from build123d import *

# Parameters (mm, degrees)
SKETCH1_W                = 151
SKETCH1_H                = 84
BOSS_EXTRUDE1_DEPTH      = 37
SKETCH3_W                = 145
SKETCH3_H                = 78
CUT_EXTRUDE3_DEPTH       = 34
SKETCH8_W                = 19
SKETCH8_H                = 14
CUT_EXTRUDE4_DEPTH       = 3
SKETCH9_W                = 19
SKETCH9_H                = 14
CUT_EXTRUDE5_DEPTH       = 3
SKETCH11_W               = 9
SKETCH11_H               = 10
CUT_EXTRUDE6_DEPTH       = 3
SKETCH12_W               = 9
SKETCH12_H               = 10
CUT_EXTRUDE7_DEPTH       = 3
BOSS_EXTRUDE2_DEPTH      = 3
BOSS_EXTRUDE2_DEPTH_BACK = 3
SKETCH19_R               = 1.5
CUT_EXTRUDE8_DEPTH       = 6
SKETCH20_W               = 3
SKETCH20_H               = 14
BOSS_EXTRUDE3_DEPTH      = 3
SKETCH21_W               = 3
SKETCH21_H               = 14
BOSS_EXTRUDE4_DEPTH      = 3
SKETCH23_W               = 16
SKETCH23_H               = 15
CUT_EXTRUDE9_DEPTH       = 3
SKETCH28_W               = 4
SKETCH28_H               = 5
BOSS_EXTRUDE5_DEPTH      = 5
MIRROR2_COPY_1_SKETCH_W  = 4
MIRROR2_COPY_1_SKETCH_H  = 5
MIRROR2_COPY_1_DEPTH     = 5


with BuildPart() as part:
    # Sketch1 → Boss-Extrude1 (new body)
    with BuildSketch(Plane.XY):
        Rectangle(SKETCH1_W, SKETCH1_H)
    extrude(amount=BOSS_EXTRUDE1_DEPTH)

    # Sketch3 → Cut-Extrude3 (cut)
    with BuildSketch(Plane.XY.offset(37)):
        Rectangle(SKETCH3_W, SKETCH3_H)
    extrude(amount=-CUT_EXTRUDE3_DEPTH, mode=Mode.SUBTRACT)

    # Sketch8 → Cut-Extrude4 (cut)
    with BuildSketch(Plane.ZY.offset(75.5)):
        with Locations((27.5, -24)):
            Rectangle(SKETCH8_W, SKETCH8_H)
    extrude(amount=-CUT_EXTRUDE4_DEPTH, mode=Mode.SUBTRACT)

    # Sketch9 → Cut-Extrude5 (cut)
    with BuildSketch(Plane.ZY.offset(75.5)):
        with Locations((27.5, -6)):
            Rectangle(SKETCH9_W, SKETCH9_H)
    extrude(amount=-CUT_EXTRUDE5_DEPTH, mode=Mode.SUBTRACT)

    # Sketch11 → Cut-Extrude6 (cut)
    with BuildSketch(Plane(origin=(75.5, 0, 0), x_dir=(0, 0, -1), z_dir=(1, 0, 0))):
        with Locations((-7.5, 32)):
            Rectangle(SKETCH11_W, SKETCH11_H)
    extrude(amount=-CUT_EXTRUDE6_DEPTH, mode=Mode.SUBTRACT)

    # Sketch12 → Cut-Extrude7 (cut)
    with BuildSketch(Plane(origin=(75.5, 0, 0), x_dir=(0, 0, -1), z_dir=(1, 0, 0))):
        with Locations((-7.5, -26)):
            Rectangle(SKETCH12_W, SKETCH12_H)
    extrude(amount=-CUT_EXTRUDE7_DEPTH, mode=Mode.SUBTRACT)

    # Sketch16 → Boss-Extrude2 (add, two sides)
    with BuildSketch(Plane.XY.offset(18)) as boss_extrude2_sk:
        with BuildLine():
            Line((75.5, 6), (75.5, -8.461119278))
            ThreePointArc((75.5, -8.461119278), (82.730559639, -1.230559639), (75.5, 6))
        make_face()
    extrude(amount=BOSS_EXTRUDE2_DEPTH)
    extrude(boss_extrude2_sk.sketch, amount=-BOSS_EXTRUDE2_DEPTH_BACK)

    # Sketch19 → Cut-Extrude8 (cut)
    with BuildSketch(Plane.XY.offset(21)):
        with Locations((79, -1)):
            Circle(SKETCH19_R)
    extrude(amount=-CUT_EXTRUDE8_DEPTH, mode=Mode.SUBTRACT)

    # Sketch20 → Boss-Extrude3 (add)
    with BuildSketch(Plane.ZY.offset(75.5)):
        with Locations((35.5, -6)):
            Rectangle(SKETCH20_W, SKETCH20_H)
    extrude(amount=-BOSS_EXTRUDE3_DEPTH)

    # Sketch21 → Boss-Extrude4 (add)
    with BuildSketch(Plane.ZY.offset(75.5)):
        with Locations((35.5, -24)):
            Rectangle(SKETCH21_W, SKETCH21_H)
    extrude(amount=-BOSS_EXTRUDE4_DEPTH)

    # Sketch23 → Cut-Extrude9 (cut)
    with BuildSketch(Plane.ZY.offset(75.5)):
        with Locations((26, 10.5)):
            Rectangle(SKETCH23_W, SKETCH23_H)
    extrude(amount=-CUT_EXTRUDE9_DEPTH, mode=Mode.SUBTRACT)

    # Sketch28 → Boss-Extrude5 (add)
    with BuildSketch(Plane.ZY.offset(-72.5)):
        with Locations((32, -36.5)):
            Rectangle(SKETCH28_W, SKETCH28_H)
    boss_extrude5 = extrude(amount=BOSS_EXTRUDE5_DEPTH)

    # Mirror1: Boss-Extrude5 across plane
    add(boss_extrude5.mirror(Plane.ZX))

    # Mirror2: Boss-Extrude5 across plane
    add(boss_extrude5.mirror(Plane(origin=(0, 0, 0), x_dir=(0, 0, 1), z_dir=(1, 0, 0))))

    # Mirror2 copy 1 sketch → Mirror2 copy 1 (add)
    with BuildSketch(Plane(origin=(-72.5, 0, 0), x_dir=(0, 0, 1), z_dir=(1, 0, 0))):
        with Locations((32, -36.5)):
            Rectangle(MIRROR2_COPY_1_SKETCH_W, MIRROR2_COPY_1_SKETCH_H)
    extrude(amount=MIRROR2_COPY_1_DEPTH)


solid = part.part
Design review of the part built by this model. Coordinates are the model's own, in mm. A direction names the side the tool comes from. Round coordinates to 2 decimals unless told otherwise and drop trailing zeros. Loops run counter-clockwise (first coordinate to the right, second up) from the corner with the lowest first, then second, coordinate; pieces in that order, holes last. Notation, with made-up numbers: (-4, 32.5) - (13, 32.5) arc R15 ccw to (13, 41.5) - close; hole circle Ø5 at (70.5, 17.25). An arc over 180 degrees is marked (long way). One line per item, written item: value. Start each with the question number.
1) Consider section A-A on z = 32. Give the boundary of the cut face in (x, y).
2) Consider section C-C on y = -1. Give the boundary of the cut face in (x, z).
3) For faces 1 (the flat face through (-74, -31, 26)), 2 (the flat face through (70, -34, 32)), 3 (the flat face through (70, 37, 30)), list the 3-axis set-ups (+Z, -Z, +X, -X, +Y, -Y) from which the entire face can be reached by the end or side of a thin tool; tool diameter is ignored.
4) To check wall thickness, follow L1, parallel to Y at x = -26, z = 15; L2, parallel to X at y = -38, z = 32; L3, parallel to X at y = 21.5, z = 7. State the ranges of each line that lie inside material, in increasing order. Write a range as from..to.
5) Consider section B-B on x = 69. Give the boundary of the cut face in (y, z), then the cut area to 3 significant figures.
6) Draft analysis for pull direction X (two halves, no side actions). For faces 4 (the flat face through (74, 32, 12)), 5 (the flat face through (-67.5, -36, 32)), 6 (the cylindrical face through (82.73, -1.39, 18.04)), 7 (the flat face through (-70, 37, 34)), state which applies: +X half, -X half, draft (parallel to the pull), parting line (faces both ways), or undercut.
7) Consider section D-D on x = 21.5. Give the boundary of the cut face in (y, z).
8) Insertion check: pin 1 Ø4 at (x, y) = (-18.5, 18) entering from -Z; pin 2 Ø1.5 at (x, y) = (-39.5, -7) entering from +Z; pin 3 Ø1.2 at (y, z) = (-36.5, 33) entering from +X; pin 4 Ø1.5 at (x, y) = (69.5, 36) entering from +Z. Each pin has a flat end and moves straight along its axis. Give the tip position at first contact, or say it passes through.
Reported:
1. outline: (-75.5, -42) - (75.5, -42) - (75.5, 42) - (-75.5, 42) - (-75.5, 18) - (-72.5, 18) - (-72.5, 34) - (-67.5, 34) - (-67.5, 39) - (67.5, 39) - (67.5, 34) - (72.5, 34) - (72.5, -34) - (67.5, -34) - (67.5, -39) - (-67.5, -39) - (-67.5, -34) - (-72.5, -34) - (-72.5, -31) - (-75.5, -31) - close; (-75.5, -17) - (-72.5, -17) - (-72.5, -13) - (-75.5, -13) - close; (-75.5, 1) - (-72.5, 1) - (-72.5, 3) - (-75.5, 3) - close
2. outline: (-75.5, 0) - (75.5, 0) - (75.5, 15) - (77.5, 15) - (77.5, 21) - (75.5, 21) - (75.5, 37) - (72.5, 37) - (72.5, 3) - (-72.5, 3) - (-72.5, 18) - (-75.5, 18) - close; (-75.5, 34) - (-72.5, 34) - (-72.5, 37) - (-75.5, 37) - close; (80.5, 15) - (82.73, 15) - (82.73, 21) - (80.5, 21) - close
3. face 1: -X
3. face 2: +Z
3. face 3: none
4. L1: y = -42..-39, 39..42
4. L2: x = -75.5..-67.5, 67.5..75.5
4. L3: x = -75.5..-72.5, 72.5..75.5
5. outline: (-42, 0) - (42, 0) - (42, 37) - (39, 37) - (39, 34) - (34, 34) - (34, 30) - (39, 30) - (39, 3) - (-39, 3) - (-39, 30) - (-34, 30) - (-34, 34) - (-39, 34) - (-39, 37) - (-42, 37) - close
5. area: 496 mm^2
6. face 4: draft
6. face 5: undercut
6. face 6: +X half
6. face 7: undercut
7. outline: (-42, 0) - (42, 0) - (42, 37) - (39, 37) - (39, 3) - (-39, 3) - (-39, 37) - (-42, 37) - close
8. pin 1: stops at z = 0
8. pin 2: stops at z = 3
8. pin 3: stops at x = 75.5
8. pin 4: stops at z = 34
